Check sheet for the modelled part. Datum: model origin and axes. Units: mm. A direction names the side the tool comes from. Round coordinates to 2 decimals unless told otherwise and drop trailing zeros. Loops run counter-clockwise (first coordinate to the right, second up) from the corner with the lowest first, then second, coordinate; pieces in that order, holes last. Notation, with made-up numbers: (78.25, 35) -> (90.25, 35) arc R28 ccw to (90.25, 53) -> close; hole circle Ø8 at (86.25, 27). An arc over 180 degrees is marked (long way). Use one line per item in the form item = value. Start each with the question number.
(1) Set-up check for faces 4 (the flat face through (-5.68, -3.82, 0.51)), 5 (the flat face through (-3.172, -9.239, 23.604)), 6 (the flat face through (5.5, -7, 12)): record each of +Z, -Z, +X, -X, +Y, -Y from which the full face is reachable in a straight line by a thin tool's end or side.
(2) Sectioned sample at B-B (z = 12). State how many separate pieces and enclosed holes the cut face has, and give its area (3 significant figures).
(3) Draft check along Y on faces 1 (the cylindrical face through (14.04, -14.05, 12.13)), 2 (the cylindrical face through (14.04, 11.85, 0.9)), 3 (the flat face through (-3.932, 9.149, 11.846)). Enter one of: released by +Y, released by -Y, zero draft, split by the parting line, or undercut.
(4) Material ranges on probe 1 along Y at (x, z) = (0, 14.5); probe 2 along Y at (x, z) = (2.75, 2.25); probe 3 along Z at (x, y) = (8.5, 0), recorded low to high. Write a range as [from, to].
(5) Sectioned sample at A-A (y = 0). Record the cut outline in (x, z), and give its area (3 significant figures).
(6) Go/stop test with flat-tipped pins: pin 1 (5.5 mm diameter, centred on y = 0, z = 12, fed in from -X); pin 2 (3 mm diameter, centred on y = 29, z = 21.5, fed in from -X); pin 3 (0.5 mm diameter, centred on x = 7.5, z = 7, fed in from +Y); pin 4 (3 mm diameter, centred on x = -2, y = 40.5, fed in from -Z). Record where each tip stops, or that it passes through.
from build123d import *

# Parameters (mm, degrees)
BOSS_EXTRUDE1_DEPTH = 24
SKETCH4_R           = 6.5
BOSS_EXTRUDE2_DEPTH = 24
SKETCH3_R           = 3
CUT_EXTRUDE1_DEPTH  = 30.899298428
FILLET1_R           = 3
CHAMFER1_SIZE       = 1


with BuildPart() as part:
    # Sketch1 → Boss-Extrude1 (new body)
    with BuildSketch(Plane.XY):
        Polygon((0, 15), (14.899298428, 15), (14.899298428, -14.949649214), (-15, -14.949649214), (-15, 15), align=None)
        Polygon((-9.966432809, 9.966432809), (-4.741432809, 9.966432809), (-3.1, 8.307461143), (-5.5, 8.307461143), (-5.5, 6.667461143), (-2.79, 3.957461143), (2.79, 3.957461143), (5.5, 6.667461143), (5.5, 8.307461143), (3.1, 8.307461143), (4.741432809, 9.966432809), (9.966432809, 9.966432809), (9.966432809, 4.741432809), (8.307461143, 3.1), (8.307461143, 5.5), (6.667461143, 5.5), (3.957461143, 2.79), (3.957461143, -2.79), (6.667461143, -5.5), (8.307461143, -5.5), (8.307461143, -3.1), (9.966432809, -4.741432809), (9.966432809, -9.966432809), (4.741432809, -9.966432809), (3.1, -8.307461143), (5.5, -8.307461143), (5.5, -6.667461143), (2.79, -3.957461143), (-2.79, -3.957461143), (-5.5, -6.667461143), (-5.5, -8.307461143), (-3.1, -8.307461143), (-4.741432809, -9.966432809), (-9.966432809, -9.966432809), (-9.966432809, -4.741432809), (-8.307461143, -3.1), (-8.307461143, -5.5), (-6.667461143, -5.5), (-3.957461143, -2.79), (-3.957461143, 2.79), (-6.667461143, 5.5), (-8.307461143, 5.5), (-8.307461143, 3.1), (-9.966432809, 4.741432809), align=None, mode=Mode.SUBTRACT)
    extrude(amount=BOSS_EXTRUDE1_DEPTH)

    # Sketch4 → Boss-Extrude2 (add)
    with BuildSketch(Plane(origin=(0, 0, 0), x_dir=(-1, 0, 0), z_dir=(0, 0, -1))):
        with BuildLine():
            ThreePointArc((-14.899298428, 35), (0.050350786, 49.949649214), (15, 35))
            Line((15, 35), (15, 15))
            Line((15, 15), (-14.899298428, 15))
            Line((-14.899298428, 15), (-14.899298428, 35))
        make_face()
        with Locations((0.050350786, 35)):
            Circle(SKETCH4_R, mode=Mode.SUBTRACT)
    extrude(amount=-BOSS_EXTRUDE2_DEPTH)

    # Sketch3 → Cut-Extrude1 (cut, through all)
    with BuildSketch(Plane.ZY.offset(15)):
        with Locations((12, 0)):
            Circle(SKETCH3_R)
    extrude(amount=-CUT_EXTRUDE1_DEPTH, mode=Mode.SUBTRACT)

    # Fillet1
    fillet1_edges = [part.edges().sort_by_distance(p)[0] for p in [
        (-0.050350786, -14.949649214, 24),
        (14.899298428, 10.025175393, 24),
        (-0.050350786, 49.949649214, 24),
        (-0.050350786, 49.949649214, 0),
        (14.899298428, 10.025175393, 0),
        (-0.050350786, -14.949649214, 0),
        (-15, 10.025175393, 0),
        (-15, 10.025175393, 24),
        (14.899298428, -14.949649214, 12),
        (-15, -14.949649214, 12),
    ]]
    fillet(fillet1_edges, radius=FILLET1_R)

    # Chamfer1
    chamfer1_edges = [part.edges().sort_by_distance(p)[0] for p in [
        (6.449649214, 35, 24),
        (6.449649214, 35, 0),
        (-4.3, 8.307461143, 0),
        (-3.920716405, 9.136946976, 0),
        (-7.353932809, 9.966432809, 0),
        (-9.966432809, 7.353932809, 0),
        (-9.136946976, 3.920716405, 0),
        (-8.307461143, 4.3, 0),
        (-7.487461143, 5.5, 0),
        (-5.312461143, 4.145, 0),
        (-3.957461143, 0, 0),
        (-5.312461143, -4.145, 0),
        (-7.487461143, -5.5, 0),
        (-8.307461143, -4.3, 0),
        (-9.136946976, -3.920716405, 0),
        (-9.966432809, -7.353932809, 0),
        (-7.353932809, -9.966432809, 0),
        (-3.920716405, -9.136946976, 0),
        (-4.3, -8.307461143, 0),
        (-5.5, -7.487461143, 0),
        (-4.145, -5.312461143, 0),
        (0, -3.957461143, 0),
        (4.145, -5.312461143, 0),
        (5.5, -7.487461143, 0),
        (4.3, -8.307461143, 0),
        (3.920716405, -9.136946976, 0),
        (7.353932809, -9.966432809, 0),
        (9.966432809, -7.353932809, 0),
        (9.136946976, -3.920716405, 0),
        (8.307461143, -4.3, 0),
        (7.487461143, -5.5, 0),
        (5.312461143, -4.145, 0),
        (3.957461143, 0, 0),
        (5.312461143, 4.145, 0),
        (7.487461143, 5.5, 0),
        (8.307461143, 4.3, 0),
        (9.136946976, 3.920716405, 0),
        (9.966432809, 7.353932809, 0),
        (7.353932809, 9.966432809, 0),
        (3.920716405, 9.136946976, 0),
        (4.3, 8.307461143, 0),
        (5.5, 7.487461143, 0),
        (4.145, 5.312461143, 0),
        (0, 3.957461143, 0),
        (-4.145, 5.312461143, 0),
        (-5.5, 7.487461143, 0),
        (-4.3, 8.307461143, 24),
        (-3.920716405, 9.136946976, 24),
        (-7.353932809, 9.966432809, 24),
        (-9.966432809, 7.353932809, 24),
        (-9.136946976, 3.920716405, 24),
        (-8.307461143, 4.3, 24),
        (-7.487461143, 5.5, 24),
        (-5.312461143, 4.145, 24),
        (-3.957461143, 0, 24),
        (-5.312461143, -4.145, 24),
        (-7.487461143, -5.5, 24),
        (-8.307461143, -4.3, 24),
        (-9.136946976, -3.920716405, 24),
        (-9.966432809, -7.353932809, 24),
        (-7.353932809, -9.966432809, 24),
        (-3.920716405, -9.136946976, 24),
        (-4.3, -8.307461143, 24),
        (-5.5, -7.487461143, 24),
        (-4.145, -5.312461143, 24),
        (0, -3.957461143, 24),
        (4.145, -5.312461143, 24),
        (5.5, -7.487461143, 24),
        (4.3, -8.307461143, 24),
        (3.920716405, -9.136946976, 24),
        (7.353932809, -9.966432809, 24),
        (9.966432809, -7.353932809, 24),
        (9.136946976, -3.920716405, 24),
        (8.307461143, -4.3, 24),
        (7.487461143, -5.5, 24),
        (5.312461143, -4.145, 24),
        (3.957461143, 0, 24),
        (5.312461143, 4.145, 24),
        (7.487461143, 5.5, 24),
        (8.307461143, 4.3, 24),
        (9.136946976, 3.920716405, 24),
        (9.966432809, 7.353932809, 24),
        (7.353932809, 9.966432809, 24),
        (3.920716405, 9.136946976, 24),
        (4.3, 8.307461143, 24),
        (5.5, 7.487461143, 24),
        (4.145, 5.312461143, 24),
        (0, 3.957461143, 24),
        (-4.145, 5.312461143, 24),
        (-5.5, 7.487461143, 24),
    ]]
    chamfer(chamfer1_edges, length=CHAMFER1_SIZE)


solid = part.part
Checks:
q1.face_4 = -Z
q1.face_5 = +Z
q1.face_6 = +Z, -Z
q2.separate_pieces = 2
q2.enclosed_holes = 1
q2.area = 1,390 mm2
q3.face_1 = released by -Y
q3.face_2 = zero draft
q3.face_3 = undercut
q4.probe_1 = [-14.95, -3.96], [3.96, 28.5], [41.5, 49.95]
q4.probe_2 = [-14.85, -3.96], [3.96, 29.13], [40.87, 49.59]
q4.probe_3 = [0, 9], [15, 24]
q5.outline = (-15, 3) arc R3 ccw to (-12, 0) -> (-4.96, 0) -> (-3.96, 1) -> (-3.96, 9) -> (-15, 9) -> close; (-15, 15) -> (-3.96, 15) -> (-3.96, 23) -> (-4.96, 24) -> (-12, 24) arc R3 ccw to (-15, 21) -> close; (3.96, 1) -> (4.96, 0) -> (11.9, 0) arc R3 ccw to (14.9, 3) -> (14.9, 9) -> (3.96, 9) -> close; (3.96, 15) -> (14.9, 15) -> (14.9, 21) arc R3 ccw to (11.9, 24) -> (4.96, 24) -> (3.96, 23) -> close
q5.area = 386 mm2
q6.pin_1 = through
q6.pin_2 = -15
q6.pin_3 = 48.05
q6.pin_4 = 0.16
